```python
from build123d import *

# Parameters (mm, degrees)
SKETCH2_W           = 25.4
SKETCH2_H           = 304.8
BOSS_EXTRUDE1_DEPTH = 1219.2


with BuildPart() as part:
    # Sketch2 → Boss-Extrude1 (new body)
    with BuildSketch(Plane.XY):
        Polygon((-76.2, 152.4), (-12.7, 152.4), (12.7, 152.4), (76.2, 152.4), (76.2, 190.5), (-76.2, 190.5), align=None)
        Rectangle(SKETCH2_W, SKETCH2_H)
        Polygon((12.7, -152.4), (-12.7, -152.4), (-76.2, -152.4), (-76.2, -190.5), (76.2, -190.5), (76.2, -152.4), align=None)
    extrude(amount=BOSS_EXTRUDE1_DEPTH)


solid = part.part
```
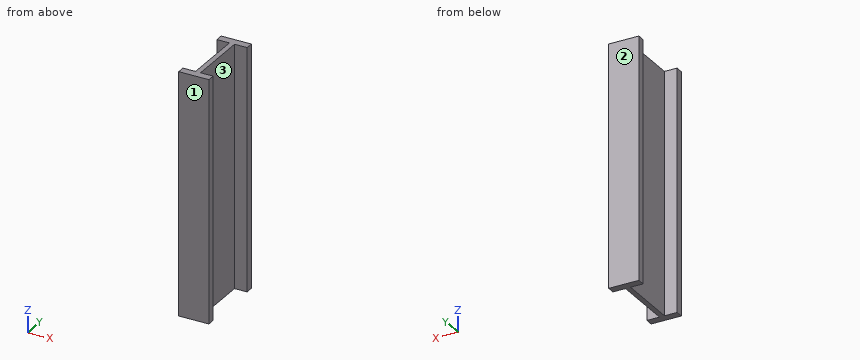
The listing builds one solid part. Answer for the finished solid, in the listing's coordinates (mm). Face numbers are marked on the shaded views. Give positions to 0.01 mm unless a question says otherwise; leave off trailing zeros. Order: outer loops, then holes, each group sorted by start corner. A loop starts at its lowest first (then second) coordinate and runs counter-clockwise, first axis right, second up. Notation, with made-up numbers: (69.25, 87) -> (89.25, 87) arc R7 ccw to (89.25, 100) -> close; hole circle Ø11 at (13, 43). An arc over 180 degrees is marked (long way). One line per item, written item: value.
1) Find section B-B, the plane z = 699.5. Determine the outline of the cut face in (x, y), plus the area to 3 significant figures.
Reported:
outline: (-76.2, -190.5) -> (76.2, -190.5) -> (76.2, -152.4) -> (12.7, -152.4) -> (12.7, 152.4) -> (76.2, 152.4) -> (76.2, 190.5) -> (-76.2, 190.5) -> (-76.2, 152.4) -> (-12.7, 152.4) -> (-12.7, -152.4) -> (-76.2, -152.4) -> close
area: 19,400 mm^2
2) Flat-ended cylindrical pins translate along their axes: P1, Ø8, axis at y = -101.5, z = 554, coming from the -X side; P2, Ø6, axis at y = -62, z = 1086, coming from the +X side. Find the tip coordinate at first contact, or state that the pin passes through.
Reported:
P1: stops at x = -12.7
P2: stops at x = 12.7
3) Find section A-A, the plane x = 60. Determine the outline of the cut face in (y, z), plus the area to 3 significant figures.
Reported:
outline: (-190.5, 0) -> (-152.4, 0) -> (-152.4, 1219.2) -> (-190.5, 1219.2) -> close; (152.4, 0) -> (190.5, 0) -> (190.5, 1219.2) -> (152.4, 1219.2) -> close
area: 92,900 mm^2
4) Find the intervals of material crossed by line 1 (Y direction, x = 54, z = 266.5); line 2 (X direction, y = -91, z = 473.5), in increasing order.
Reported:
line 1: y = -190.5 to -152.4, 152.4 to 190.5
line 2: x = -12.7 to 12.7
5) Find section C-C, the plane y = -130.5. Determine the outline of the cut face in (x, z).
Reported:
outline: (-12.7, 0) -> (12.7, 0) -> (12.7, 1219.2) -> (-12.7, 1219.2) -> close
6) Determine the mould class of the marked faces 1, 2 and 3 for opening direction Y: pulls with the +Y half, pulls with the -Y half, needs draft (parallel to the pull), parting line crosses it, or undercut.
Reported:
face 1: pulls with the -Y half
face 2: pulls with the +Y half
face 3: undercut
